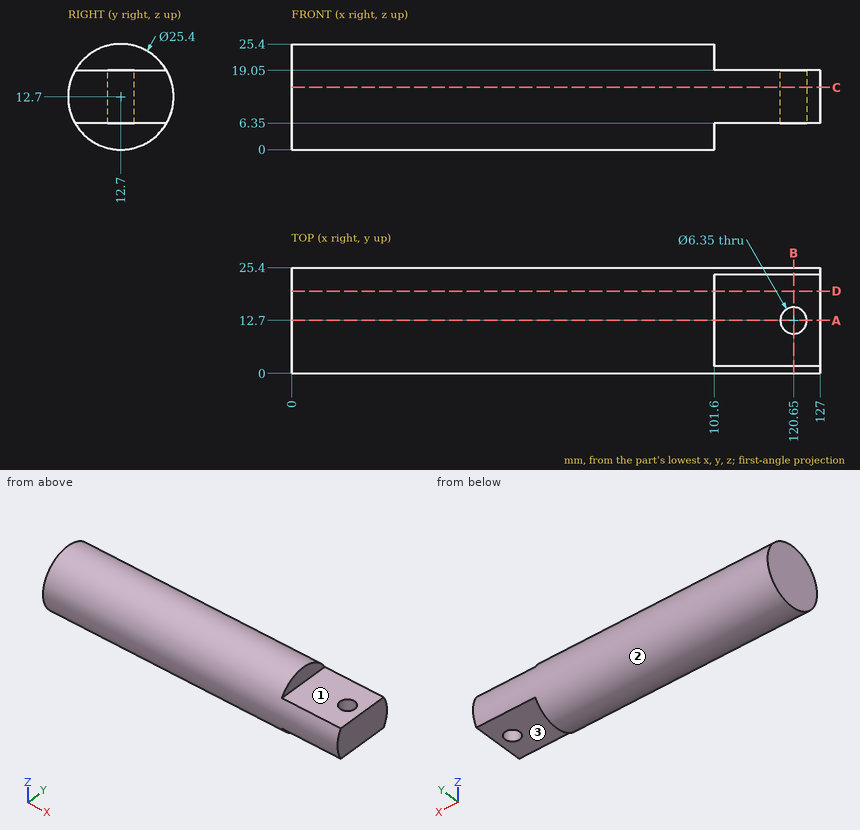
Answer from the drawing. Dimensions are ordinates in mm from the lowest x, y and z of the part. A direction names the side the tool comes from. Coordinates: 2 decimals unless noted, no trailing zeros. Order: outer loops, then holes, each group sorted by start corner. A loop starts at its lowest first (then second) coordinate and runs counter-clockwise, first axis right, second up. Notation, with made-up numbers: M 3.25,3 L 16.25,3 A18 ccw 16.25,11 Z; hole C 61.25,72.5 d1. An arc over 180 degrees is marked long. Put each result on its own line as item: value. Start each with the question number.
Item 1: Given pin 1 Ø6.5 at (x, y) = (110, 14) entering from +Z; pin 2 Ø1.9 at (y, z) = (18, 4.5) entering from +X; pin 3 Ø3 at (x, z) = (40.5, 6) entering from +Y, each flat-ended and moving along its own axis, determine where each tip first touches the part or whether it passes through.
Item 2: Section B-B, the plane x = 120.65 is taken. Determine the outline of the cut face in (y, z) (3 decimals), plus the area to 3 significant figures.
Item 3: For the marked faces 1, 2 and 3, determine the directions among +Z, -Z, +X, -X, +Y, -Y from which every point of the face is accessible in a straight line to the end or side of a thin tool.
Item 4: Section A-A, the plane y = 12.7 is taken. Determine the outline of the cut face in (x, z) (3 decimals), plus the area to 3 significant figures.
Item 5: Consider probe 1 along Y at (x, z) = (120.65, 13.25) (3 decimals); probe 2 along Y at (x, z) = (120.65, 9) (3 decimals); probe 3 along X at (y, z) = (5, 4.5). Determine where each line is inside the solid, lowest interval first. Write a range as [from, to].
Item 6: Section D-D, the plane y = 19.75 is taken. Determine the outline of the cut face in (x, z).
Item 7: Section C-C, the plane z = 15 is taken. Determine the outline of the cut face in (x, y) (3 decimals).
Computed:
1. pin 1: stops at z = 19.05
1. pin 2: stops at x = 101.6
1. pin 3: stops at y = 24.29
2. outline: M 1.701,6.35 L 9.525,6.35 L 9.525,19.05 L 1.701,19.05 A12.7 ccw Z; M 15.875,6.35 L 23.699,6.35 A12.7 ccw 23.699,19.05 L 15.875,19.05 Z
2. area: 228 mm2
3. face 1: +Z, +X, +Y, -Y
3. face 2: +X, -X
3. face 3: -Z, +X, +Y, -Y
4. outline: M 0,0 L 101.6,0 L 101.6,6.35 L 117.475,6.35 L 117.475,19.05 L 101.6,19.05 L 101.6,25.4 L 0,25.4 Z; M 123.825,6.35 L 127,6.35 L 127,19.05 L 123.825,19.05 Z
4. area: 2,820 mm2
5. probe 1: y = [0.012, 9.525], [15.875, 25.388]
5. probe 2: y = [0.551, 9.525], [15.875, 24.849]
5. probe 3: x = [0, 101.6]
6. outline: M 0,2.14 L 101.6,2.14 L 101.6,6.35 L 127,6.35 L 127,19.05 L 101.6,19.05 L 101.6,23.26 L 0,23.26 Z
7. outline: M 0,0.21 L 127,0.21 L 127,25.19 L 0,25.19 Z; hole C 120.65,12.7 d6.35
